Can you work these out from the model? Positions are in its coordinate system, mm. A direction names the side the tool comes from. Give positions to 0.01 mm unless a question says otherwise; leave off trailing zeros. Loops run counter-clockwise (first coordinate to the right, second up) from the corner with the lowest first, then second, coordinate; pieces in that order, holes last. Notation, with made-up numbers: (46.5, 63) -> (73.5, 63) arc R36 cw to (73.5, 97) -> close; hole circle Ø3 at (89, -25). An arc over 180 degrees is marked (long way). Use CSV: the item, a comma, the result in double quotes.
from build123d import *

# Parameters (mm, degrees)
F1_DEPTH = 15
F2_R     = 0.2
F3_R     = 1.5
F4_DEPTH = 10
F5_R     = 1.5
F6_DEPTH = 4


with BuildPart() as f1:
    # F0 (on Front) → F1 (new body)
    with BuildSketch(Plane.XZ):
        Polygon((1.0103629711, -1.75), (2.0207259422, 0), (1.0103629711, 1.75), (-1.0103629711, 1.75), (-2.0207259422, 0), (-1.0103629711, -1.75), align=None)
    extrude(amount=F1_DEPTH)

    # F2
    f2_edges = [f1.edges().sort_by_distance(p)[0] for p in [
        (-1.010363, -7.5, 1.75),
        (1.010363, -7.5, 1.75),
        (2.020726, -7.5, 0),
        (1.010363, -7.5, -1.75),
        (-1.010363, -7.5, -1.75),
        (-2.020726, -7.5, 0),
    ]]
    fillet(f2_edges, radius=F2_R)

    # F3 (on face) → F4 (cut)
    with BuildSketch(Plane.XZ.offset(15)):
        Circle(F3_R)
    extrude(amount=-F4_DEPTH, mode=Mode.SUBTRACT)

    # F5 (on face) → F6 (join)
    with BuildSketch(Plane(origin=(0, 0, 0), x_dir=(-1, 0, 0), z_dir=(0, 1, 0))):
        Circle(F5_R)
    extrude(amount=F6_DEPTH)


solid = f1.part
(1) Which directions (+Z, -Z, +X, -X, +Y, -Y) give clear straight access to the entire face, cutting with the end or side of a thin tool? Please do faces 5 (the face through (1.5, 1.97, 0.07)), 6 (the face through (-1.5, -7.4, -0.9)).
Answer sheet:
face 5,"+Y"
face 6,"-Z, -X, +Y, -Y"
(2) If we section it at B-B, the plane x = 0: Write out the boundary of the cut face in (y, z).
Answer sheet:
outline,"(-15, -1.75) -> (0, -1.75) -> (0, -1.5) -> (4, -1.5) -> (4, 1.5) -> (0, 1.5) -> (0, 1.75) -> (-15, 1.75) -> (-15, 1.5) -> (-5, 1.5) -> (-5, -1.5) -> (-15, -1.5) -> close"
(3) If we section it at D-D, the plane y = 1.25: Write out the boundary of the cut face in (x, z).
Answer sheet:
outline,"circle Ø3 at (0, 0)"
(4) Will this pin go through, and if not, where does the flat tip stop? pin 1 Ø1.5 at (y, z) = (-5, 1) entering from -X.
Answer sheet:
pin 1,"stops at x = -1.88"
(5) If we section it at A-A, the plane y = -4.75: Write out the boundary of the cut face in (x, z).
Answer sheet:
outline,"(-1.96, -0.1) -> (-1.07, -1.65) arc R0.2 ccw to (-0.89, -1.75) -> (0.89, -1.75) arc R0.2 ccw to (1.07, -1.65) -> (1.96, -0.1) arc R0.2 ccw to (1.96, 0.1) -> (1.07, 1.65) arc R0.2 ccw to (0.89, 1.75) -> (-0.89, 1.75) arc R0.2 ccw to (-1.07, 1.65) -> (-1.96, 0.1) arc R0.2 ccw to start"
(6) If I drill on L1, parallel to Z at x = 0, y = -10.5; L2, parallel to Y at x = -0.9, z = -1.5; L3, parallel to X at y = -12.75, z = -0.1, over which ranges is the centre line in solid material (lowest first)? Write a range as from..to.
Answer sheet:
L1,"z = -1.75..-1.5, 1.5..1.75"
L2,"y = -15..0"
L3,"x = -1.96..-1.5, 1.5..1.96"
(7) We'd pull the mould along Z, two halves only. Please class faces 1 (the face through (-1.5, -10.07, 0.07)), 2 (the face through (1.5, -7.4, -0.9)), 3 (the face through (-1.5, -7.4, 0.9)), 4 (the face through (0, -5, 0)): released by +Z, released by -Z, zero draft, split by the parting line, or undercut.
Answer sheet:
face 1,"undercut"
face 2,"released by -Z"
face 3,"released by +Z"
face 4,"undercut"
(8) If we section it at C-C, the plane y = -10.5: Write out the boundary of the cut face in (x, z).
Answer sheet:
outline,"(-1.96, -0.1) -> (-1.07, -1.65) arc R0.2 ccw to (-0.89, -1.75) -> (0.89, -1.75) arc R0.2 ccw to (1.07, -1.65) -> (1.96, -0.1) arc R0.2 ccw to (1.96, 0.1) -> (1.07, 1.65) arc R0.2 ccw to (0.89, 1.75) -> (-0.89, 1.75) arc R0.2 ccw to (-1.07, 1.65) -> (-1.96, 0.1) arc R0.2 ccw to start; hole circle Ø3 at (0, 0)"
